Study the drawing (mm; zero at the part's minimum x, y, z) and answer. Coordinates: 2 decimals unless noted, no trailing zeros. Loops run counter-clockwise (first coordinate to the right, second up) from the corner with the lowest first, then second, coordinate; pieces in that order, holes last. Notation, with made-up numbers: (68, 67) - (88, 67) arc R13 ccw to (88, 72) - close; hole circle Ø4 at (-19, 49). An arc over 180 degrees is marked (long way). One line per item, written item: value. Start each with the question number.
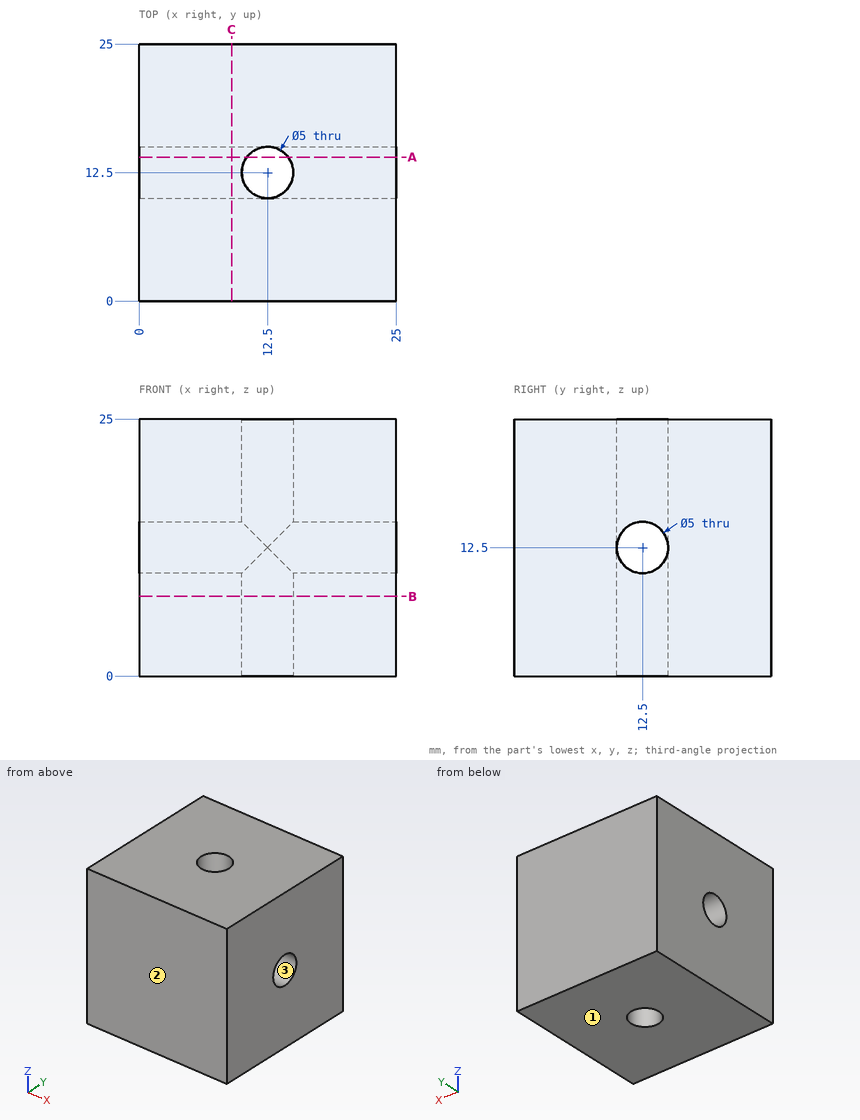
1) A flat-ended cylindrical pin translates along its axis: P1, Ø4.5, axis at x = 12.5, y = 12.5, coming from the +Z side. Find the tip coordinate at first contact, or state that the pin passes through.
2) A straight line is drawn through the part: L1, parallel to Y at x = 12.5, z = 5.75. Find the intervals that lie inside material, in ascending order.
3) Section A-A, the plane y = 14 is taken. Determine the outline of the cut face in (x, z).
4) Determine the mould class of the marked faces 1, 2 and 3 for opening direction Y: released by +Y, released by -Y, zero draft, split by the parting line, or undercut.
5) Section B-B, the plane z = 7.75 is taken. Determine the outline of the cut face in (x, y), and give its area (3 significant figures).
Answer below:
1. P1: through
2. L1: 0 to 10, 15 to 25
3. outline: (0, 0) - (10.5, 0) - (10.5, 10.5) - (0, 10.5) - close; (0, 14.5) - (10.5, 14.5) - (10.5, 25) - (0, 25) - close; (14.5, 0) - (25, 0) - (25, 10.5) - (14.5, 10.5) - close; (14.5, 14.5) - (25, 14.5) - (25, 25) - (14.5, 25) - close
4. face 1: zero draft
4. face 2: released by -Y
4. face 3: undercut
5. outline: (0, 0) - (25, 0) - (25, 25) - (0, 25) - close; hole circle Ø5 at (12.5, 12.5)
5. area: 605 mm2
